Check sheet for the modelled part. Datum: model origin and axes. Units: mm. Face numbers are marked on the shaded views. A direction names the side the tool comes from. Coordinates: 2 decimals unless noted, no trailing zeros. Write each loop counter-clockwise with the first axis right and the second up, starting at its lowest first coordinate (ties: lowest second). Pieces come first, ordered by that corner, then holes. Notation, with made-up numbers: (0, 77.25) - (55, 77.25) arc R19 ccw to (55, 111.25) - close; hole circle Ø9 at (72, 12). An arc over 180 degrees is marked (long way). Answer as CSV lines item,"result". Start each with the question number.
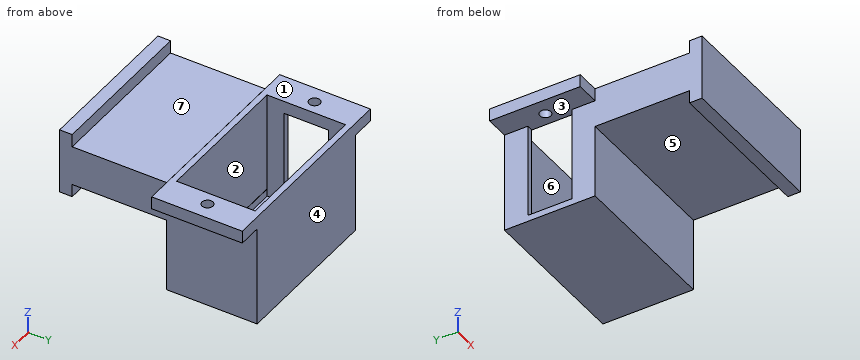
from build123d import *

# Parameters (mm, degrees)
F0_W          = 24.8
F0_H          = 18
F0_W_2        = 22.8
F0_H_2        = 16
F1_DEPTH      = 6.2
F1_DEPTH_BACK = 6.2
F2_W          = 24.8
F2_H          = 18
F3_DEPTH      = 1
F5_W          = 22.8
F5_H          = 12.48
F6_DEPTH      = 15.8
F7_W          = 9.005438
F7_H          = 7
F8_DEPTH      = 17
F10_W         = 32.3
F10_H         = 14.4
F10_W_2       = 22.8
F10_H_2       = 12.48
F11_DEPTH     = 2
F12_R         = 0.875
F13_DEPTH     = 25
F15_DEPTH     = 24.8


with BuildPart() as f1:
    # F0 (on Front) → F1 (new body, two sides)
    with BuildSketch(Plane.XZ) as f1_sk:
        with Locations((-17.722324, 14.856741)):
            Rectangle(F0_W, F0_H)
        with Locations((-17.722324, 14.856741)):
            Rectangle(F0_W_2, F0_H_2, mode=Mode.SUBTRACT)
    extrude(amount=F1_DEPTH)
    extrude(f1_sk.sketch, amount=-F1_DEPTH_BACK)

    # F2 (on face) → F3 (join)
    with BuildSketch(Plane.XZ.offset(6.2)):
        with Locations((-17.722324, 14.856741)):
            Rectangle(F2_W, F2_H)
    extrude(amount=F3_DEPTH)

    # F4: F1 across plane


with BuildPart() as f1_1:
    add(f1.part)
    add(f1.part.mirror(Plane.XZ))

    # F5 (on face) → F6 (cut)
    with BuildSketch(Plane.XY.offset(23.856741)):
        with Locations((-17.722324, 0)):
            Rectangle(F5_W, F5_H)
    extrude(amount=-F6_DEPTH, mode=Mode.SUBTRACT)

    # F7 (on face) → F8 (cut, through all)
    with BuildSketch(Plane.XY.offset(23.856741)):
        with Locations((-31.029159, 0)):
            Rectangle(F7_W, F7_H)
    extrude(amount=-F8_DEPTH, mode=Mode.SUBTRACT)

    # F10 (on face) → F11 (join)
    with BuildSketch(Plane.XY.offset(23.856741)):
        with Locations((-17.722324, 0)):
            Rectangle(F10_W, F10_H)
        with Locations((-17.722324, 0)):
            Rectangle(F10_W_2, F10_H_2, mode=Mode.SUBTRACT)
    extrude(amount=-F11_DEPTH)

    # F12 (on face) → F13 (cut)
    with BuildSketch(Plane.XY.offset(23.856741)):
        with Locations((-31.222324, 0)):
            Circle(F12_R)
        with Locations((-4.222324, 0)):
            Circle(F12_R)
    extrude(amount=-F13_DEPTH, mode=Mode.SUBTRACT)

    # F14 (on face) → F15 (join, through all)
    with BuildSketch(Plane.YZ.offset(-5.322324)):
        Polygon((-7.2, 21.856741), (-7.2, 23.879181), (-22.2, 23.879181), (-22.2, 25.934181), (-24.2, 25.934181), (-24.2, 15.484181), (-22.2, 15.484181), (-22.2, 17.539181), (-7.2, 17.539181), align=None)
    extrude(amount=-F15_DEPTH)


solid = f1_1.part
(1) Tool access check on the marked faces 1, 2, 3, 4 and 5. Record the directions out of +Z, -Z, +X, -X, +Y, -Y that give a thin tool (end or side, any length) a straight path to the whole face; none if there is none.
(2) Cross-section at D-D on y = -19. Record the boundary of the cut face in (x, z), plus the area to 3 significant figures.
(3) Release check for a two-part mould opening along X. For the marked faces 6 and 7 record: pulls with the +X half, pulls with the -X half, needs draft (parallel to the pull), parting line crosses it, or undercut.
(4) Go/stop test with flat-tipped pins: P1, Ø0.6, axis at x = -21.5, z = 25, coming from the +Y side; P2, Ø6, axis at y = -15.5, z = 17.5, coming from the +X side; P3, Ø2, axis at x = -31, z = 23.5, coming from the -Y side; P4, Ø2, axis at x = -3.5, z = 22.5, coming from the -Y side. Record where each tip stops, or that it passes through.
(5) Cross-section at C-C on z = 15. Record the boundary of the cut face in (x, y), plus the area to 3 significant figures.
(6) Cross-section at A-A on y = 0. Record the boundary of the cut face in (x, z).
(7) Material ranges on probe 1 along Y at (x, z) = (-10, 13); probe 2 along X at (y, z) = (6, 12.5); probe 3 along Z at (x, y) = (-6, -15.5), recorded low to high. Write a range as from..to.
Checked values:
1,face 1,"+Z, +X, -X, +Y"
1,face 2,"+Z"
1,face 3,"-X"
1,face 4,"+Z, -Z, +X, -X, +Y"
1,face 5,"-Z, +X, -X"
2,outline,"(-30.12, 17.54) - (-5.32, 17.54) - (-5.32, 23.88) - (-30.12, 23.88) - close"
2,area,"157 mm^2"
3,face 6,"undercut"
3,face 7,"needs draft"
4,P1,"y = -22.2"
4,P2,"x = -5.32"
4,P3,"y = -24.2"
4,P4,"y = -7.2"
5,outline,"(-30.12, -7.2) - (-5.32, -7.2) - (-5.32, 7.2) - (-30.12, 7.2) - (-30.12, 3.5) - (-29.12, 3.5) - (-29.12, 6.24) - (-6.32, 6.24) - (-6.32, -6.24) - (-29.12, -6.24) - (-29.12, -3.5) - (-30.12, -3.5) - close"
5,area,"65.6 mm^2"
6,outline,"(-33.87, 21.86) - (-32.1, 21.86) - (-32.1, 23.86) - (-33.87, 23.86) - close; (-30.35, 21.86) - (-29.12, 21.86) - (-29.12, 23.86) - (-30.35, 23.86) - close; (-30.12, 5.86) - (-5.32, 5.86) - (-5.32, 21.86) - (-5.1, 21.86) - (-5.1, 23.86) - (-6.32, 23.86) - (-6.32, 6.86) - (-30.12, 6.86) - close; (-3.35, 21.86) - (-1.57, 21.86) - (-1.57, 23.86) - (-3.35, 23.86) - close"
7,probe 1,"-7.2..-6.24, 6.24..7.2"
7,probe 2,"-30.12..-29.12, -6.32..-5.32"
7,probe 3,"17.54..23.88"
